```python
from build123d import *

# Parameters (mm, degrees)
F0_W     = 40
F0_H     = 40
F0_R     = 3
F0_R_2   = 11.2
F1_DEPTH = 10
F0_R_3   = 6.15
F2_DEPTH = 3
F3_R     = 5


with BuildPart() as f1:
    # F0 (on Top) → F1 (new body)
    with BuildSketch(Plane.XY):
        Rectangle(F0_W, F0_H)
        with Locations((-13.5, -13.5)):
            Circle(F0_R, mode=Mode.SUBTRACT)
        with Locations((13.5, -13.5)):
            Circle(F0_R, mode=Mode.SUBTRACT)
        with Locations((-13.5, 13.5)):
            Circle(F0_R, mode=Mode.SUBTRACT)
        Circle(F0_R_2, mode=Mode.SUBTRACT)
        with Locations((13.5, 13.5)):
            Circle(F0_R, mode=Mode.SUBTRACT)
    extrude(amount=F1_DEPTH)

    # F0 (on Top) → F2 (join)
    with BuildSketch(Plane.XY):
        Circle(F0_R_2)
        Circle(F0_R_3, mode=Mode.SUBTRACT)
    extrude(amount=F2_DEPTH)

    # F3
    f3_edges = [f1.edges().sort_by_distance(p)[0] for p in [
        (-20, -20, 5),
        (20, -20, 5),
        (20, 20, 5),
        (-20, 20, 5),
    ]]
    fillet(f3_edges, radius=F3_R)


solid = f1.part
```
The model under review builds one solid part; all positions refer to its coordinate system, in mm. A direction names the side the tool comes from. Round coordinates to 2 decimals unless told otherwise and drop trailing zeros. Loops run counter-clockwise (first coordinate to the right, second up) from the corner with the lowest first, then second, coordinate; pieces in that order, holes last. Notation, with made-up numbers: M 44.5,79.25 L 50.5,79.25 A25 cw 50.5,100.25 Z; hole C -15.5,-7.5 d7. An arc over 180 degrees is marked long. Answer as a JSON object with one key per item and string values.
(1) Take a section at C-C on z = 5.75. Give the boundary of the cut face in (x, y), and give its area (3 significant figures).
Resolved:
{"outline": "M -20,-15 A5 ccw -15,-20 L 15,-20 A5 ccw 20,-15 L 20,15 A5 ccw 15,20 L -15,20 A5 ccw -20,15 Z; hole C -13.5,-13.5 d6; hole C -13.5,13.5 d6; hole C 0,0 d22.4; hole C 13.5,-13.5 d6; hole C 13.5,13.5 d6", "area": "1,070 mm²"}
(2) Draft analysis for pull direction X (two halves, no side actions). For faces 3 (the cylindrical face through (-1.333, -6.004, 1.479)), 4 (the flat face through (9, 9, 10)), 5 (the cylindrical face through (-19, 18, 5)), state which applies: released by +X, released by -X, zero draft, split by the parting line, or undercut.
Resolved:
{"face 3": "undercut", "face 4": "zero draft", "face 5": "released by -X"}
(3) Tool access review of faces 1 (the flat face through (5, -5, 3)), 2 (the flat face through (0, -20, 5)): name each direction out of +Z, -Z, +X, -X, +Y, -Y from which nothing blocks a thin tool from reaching the whole face with its end or side.
Resolved:
{"face 1": "+Z", "face 2": "+Z, -Z, +X, -X, -Y"}
(4) Take a section at D-D on x = 0. Give the boundary of the cut face in (y, z), and give its area (3 significant figures).
Resolved:
{"outline": "M -20,0 L -6.15,0 L -6.15,3 L -11.2,3 L -11.2,10 L -20,10 Z; M 6.15,0 L 20,0 L 20,10 L 11.2,10 L 11.2,3 L 6.15,3 Z", "area": "206 mm²"}
(5) Take a section at A-A on x = -13.5. Give the boundary of the cut face in (y, z), and give its area (3 significant figures).
Resolved:
{"outline": "M -20,0 L -16.5,0 L -16.5,10 L -20,10 Z; M -10.5,0 L 10.5,0 L 10.5,10 L -10.5,10 Z; M 16.5,0 L 20,0 L 20,10 L 16.5,10 Z", "area": "280 mm²"}
(6) Clearance check with flat-ended pins moving along their axes: P1, Ø7, axis at x = -13.5, y = -13.5, coming from the -Z side; P2, Ø5.5, axis at x = 13.5, y = -13.5, coming from the -Z side; P3, Ø6.5, axis at x = 0, y = 4.5, coming from the +Z side. State where each tip first meets the part, or that it passes through.
Resolved:
{"P1": "z = 0", "P2": "through", "P3": "z = 3"}
(7) To check wall thickness, follow line 1 along Y through (x, z) = (-13.5, 7.5); line 2 along Y through (x, z) = (0, 1.05); line 3 along Y through (x, z) = (0, 7.75). State the ranges of each line that lie inside material, in increasing order.
Resolved:
{"line 1": "-20 to -16.5, -10.5 to 10.5, 16.5 to 20", "line 2": "-20 to -6.15, 6.15 to 20", "line 3": "-20 to -11.2, 11.2 to 20"}
